Could you check a few things on this model? Use its own coordinates, in mm. A direction names the side the tool comes from. Give positions to 0.01 mm unless a question says otherwise; leave off trailing zeros. Loops run counter-clockwise (first coordinate to the right, second up) from the corner with the lowest first, then second, coordinate; pieces in that order, holes last. Notation, with made-up numbers: M 64,-16 L 110,-16 A27 ccw 110,23 Z; hole C 43.5,29 d4. An arc over 180 degrees is marked long. Return JSON: item names as keys, results as strings. Group by question number.
1. Please list where these lines run through material, in increasing order: line 1 (X direction, y = -2.65, z = 0.5) (1 decimal); line 2 (Z direction, x = -33, y = -0.45); line 3 (X direction, y = -1.6, z = -7) (1 decimal).
2. If we section it at B-B (y = -2.9): Write out the boundary of the cut face in (x, z) (1 decimal).
3. If we section it at D-D (z = -11): Write out the boundary of the cut face in (x, y) (1 decimal), plus the area to 3 significant figures.
4. For faces 1 (the flat face through (-21.688, -2, 0)), 2 (the flat face through (-1, -3.5, 1)), which set-ups out of +Z, -Z, +X, -X, +Y, -Y let a thin tool reach every point of the face, with its end or its side?
5. If we mould it in two halves opening along X, with no side actions, what happens to faces 3 (the flat face through (-1, 0, 1)), 4 (the cylindrical face through (-64.621, -1.726, 41.074)), 5 (the cylindrical face through (57.86, -1.73, 7.81))? For each: +X half, -X half, draft (parallel to the pull), parting line (faces both ways), or undercut.
6. If we section it at C-C (z = 0): Write out the boundary of the cut face in (x, y) (1 decimal), plus the area to 3 significant figures.
7. If we section it at A-A (x = -34): Write out the boundary of the cut face in (y, z), plus the area to 3 significant figures.
```python
from build123d import *

# Parameters (mm, degrees)
F0_W     = 22.75
F0_H     = 41
F0_R     = 26
F1_DEPTH = 3.5


with BuildPart() as f1:
    # F0 (on Front) → F1 (new body)
    with BuildSketch(Plane.XZ):
        with BuildLine():
            Line((-61.125, -42.5), (61.125, -42.5))
            ThreePointArc((61.125, -42.5), (64.660534, -41.035534), (66.125, -37.5))
            Line((66.125, -37.5), (66.125, 37.5))
            ThreePointArc((66.125, 37.5), (64.660534, 41.035534), (61.125, 42.5))
            Line((61.125, 42.5), (-61.125, 42.5))
            ThreePointArc((-61.125, 42.5), (-64.660534, 41.035534), (-66.125, 37.5))
            Line((-66.125, 37.5), (-66.125, -37.5))
            ThreePointArc((-66.125, -37.5), (-64.660534, -41.035534), (-61.125, -42.5))
        make_face()
        with Locations((-33.0625, 0)):
            Rectangle(F0_W, F0_H, mode=Mode.SUBTRACT)
        with Locations((33.0625, 0)):
            Circle(F0_R, mode=Mode.SUBTRACT)
    extrude(amount=F1_DEPTH)


solid = f1.part
```
Answer:
{
 "1": {"line 1": "x = -66.1 to -44.4, -21.7 to 7.1, 59.1 to 66.1", "line 2": "z = -42.5 to -20.5, 20.5 to 42.5", "line 3": "x = -66.1 to -44.4, -21.7 to 8, 58.1 to 66.1"},
 "2": {"outline": "M -66.1,-37.5 A5 ccw -61.1,-42.5 L 61.1,-42.5 A5 ccw 66.1,-37.5 L 66.1,37.5 A5 ccw 61.1,42.5 L -61.1,42.5 A5 ccw -66.1,37.5 Z; hole M -44.4,-20.5 L -21.7,-20.5 L -21.7,20.5 L -44.4,20.5 Z; hole C 33.1,0 d52"},
 "3": {"outline": "M -66.1,-3.5 L -44.4,-3.5 L -44.4,0 L -66.1,0 Z; M -21.7,-3.5 L 9.5,-3.5 L 9.5,0 L -21.7,0 Z; M 56.6,-3.5 L 66.1,-3.5 L 66.1,0 L 56.6,0 Z", "area": "218 mm²"},
 "4": {"face 1": "+Y, -Y", "face 2": "+Z, -Z, +X, -X, -Y"},
 "5": {"face 3": "draft", "face 4": "-X half", "face 5": "undercut"},
 "6": {"outline": "M -66.1,-3.5 L -44.4,-3.5 L -44.4,0 L -66.1,0 Z; M -21.7,-3.5 L 7.1,-3.5 L 7.1,0 L -21.7,0 Z; M 59.1,-3.5 L 66.1,-3.5 L 66.1,0 L 59.1,0 Z", "area": "201 mm²"},
 "7": {"outline": "M -3.5,-42.5 L 0,-42.5 L 0,-20.5 L -3.5,-20.5 Z; M -3.5,20.5 L 0,20.5 L 0,42.5 L -3.5,42.5 Z", "area": "154 mm²"}
}
